Verification items for the finished model (mm, model axes). Face numbers are marked on the shaded views. Round coordinates to 2 decimals unless told otherwise and drop trailing zeros. Loops run counter-clockwise (first coordinate to the right, second up) from the corner with the lowest first, then second, coordinate; pieces in that order, holes last. Notation, with made-up numbers: (43, 70.5) - (48, 70.5) arc R27 ccw to (48, 92.5) - close; hole circle Ø9 at (-15.5, 72.5). An arc over 180 degrees is marked (long way). Use a Markdown table: item, result. Add a question column.
```python
from build123d import *

# Parameters (mm, degrees)
ESQUISSE1_W        = 39
ESQUISSE1_H        = 27
ESQUISSE1_W_2      = 33
ESQUISSE1_H_2      = 21
BOSS_EXTRU_1_DEPTH = 1.2
ESQUISSE2_W        = 39
ESQUISSE2_H        = 27
ESQUISSE2_W_2      = 36
ESQUISSE2_H_2      = 24
BOSS_EXTRU_3_DEPTH = 3.2
ESQUISSE3_W        = 39
ESQUISSE3_H        = 27
BOSS_EXTRU_4_DEPTH = 1.2
ESQUISSE5_R        = 6
BOSS_EXTRU_6_DEPTH = 20
ESQUISSE6_R        = 7.123023745
BOSS_EXTRU_7_DEPTH = 1.5
CONG_1_R           = 1.2


with BuildPart() as part:
    # Esquisse1 → Boss.-Extru.1 (new body)
    with BuildSketch(Plane(origin=(0, 0, 0), x_dir=(1, 0, 0), z_dir=(0, 1, 0))):
        with Locations((16.5, 10.5)):
            Rectangle(ESQUISSE1_W, ESQUISSE1_H)
        with Locations((16.5, 10.5)):
            Rectangle(ESQUISSE1_W_2, ESQUISSE1_H_2, mode=Mode.SUBTRACT)
    extrude(amount=BOSS_EXTRU_1_DEPTH)

    # Esquisse2 → Boss.-Extru.3 (add)
    with BuildSketch(Plane(origin=(0, 0, 0), x_dir=(-1, 0, 0), z_dir=(0, -1, 0))):
        with Locations((-16.5, 10.5)):
            Rectangle(ESQUISSE2_W, ESQUISSE2_H)
        with Locations((-16.5, 10.5)):
            Rectangle(ESQUISSE2_W_2, ESQUISSE2_H_2, mode=Mode.SUBTRACT)
    extrude(amount=BOSS_EXTRU_3_DEPTH)

    # Esquisse3 → Boss.-Extru.4 (add)
    with BuildSketch(Plane(origin=(0, -3.2, 0), x_dir=(-1, 0, 0), z_dir=(0, -1, 0))):
        with Locations((-16.5, 10.5)):
            Rectangle(ESQUISSE3_W, ESQUISSE3_H)
    extrude(amount=BOSS_EXTRU_4_DEPTH)

    # Esquisse5 → Boss.-Extru.6 (add)
    with BuildSketch(Plane(origin=(0, -4.4, 0), x_dir=(-1, 0, 0), z_dir=(0, -1, 0))):
        with Locations(Location((-16.5, 10.5, 0), (0, 0, 90))):
            Circle(ESQUISSE5_R)
    extrude(amount=BOSS_EXTRU_6_DEPTH)

    # Esquisse6 → Boss.-Extru.7 (add)
    with BuildSketch(Plane.XZ.offset(4.4)):
        with Locations(Location((16.5, -10.5, 0), (0, 0, 270))):
            Circle(ESQUISSE6_R)
    extrude(amount=BOSS_EXTRU_7_DEPTH)

    # Congé1
    # the kernel refuses this fillet: 1.2 mm, written as the material it takes off along each edge
    with BuildSketch(Plane(origin=(16.5, -5.9, -10.5), x_dir=(0, 0, -1), z_dir=(-1, 0, 0))) as cong_1_piece_1:
        with BuildLine():
            CenterArc((5.923023745, -1.197528562), CONG_1_R, 0, 86.32212933)
            Line((6, 0), (6.001539525, 0.023950571))
            ThreePointArc((6.001539525, 0.023950571), (6.561511873, 0.024), (7.123023745, 0.024))
            Line((7.123023745, 0.024), (7.147023745, 0))
            Line((7.147023745, 0), (7.147023745, -1.197528562))
            Line((7.147023745, -1.197528562), (7.123023745, -1.197528562))
        make_face()
    revolve(axis=Axis((16.5, -5.9, -10.5), (0, -1, 0)), mode=Mode.SUBTRACT)

    # Esquisse7 → Révolution2 (revolve)
    with BuildSketch(Plane.XZ.offset(24.4)):
        with BuildLine():
            Line((3.633416396, -7.841279791), (29.203795551, -12.548265009))
            ThreePointArc((29.203795551, -12.548265009), (14.065113365, -22.979961978), (3.633416396, -7.841279791))
        make_face()
    revolve(axis=Axis((3.633416396, -24.4, -7.841279791), (0.9834761213686738, 0, -0.181037892988263)))


solid = part.part
```
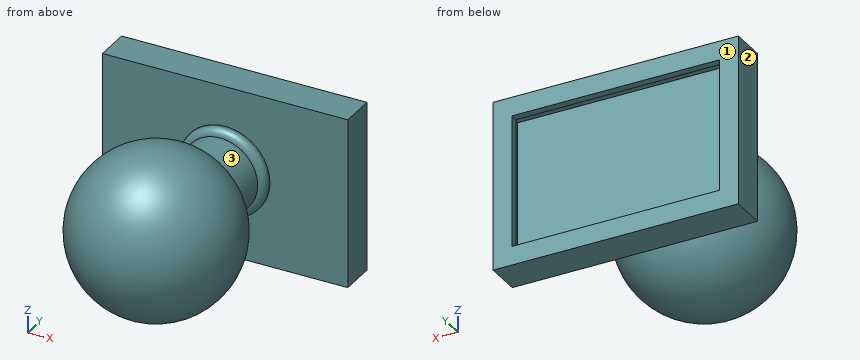
Q1. Go/stop test with flat-tipped pins: pin 1 Ø12 at (x, z) = (3, -2) entering from -Y; pin 2 Ø4 at (x, z) = (28.5, -13.5) entering from +Y; pin 3 Ø3 at (y, z) = (-29, -19.5) entering from +X. Record where each tip stops, or that it passes through.
Q2. Thickness scan on line 1 along X through (y, z) = (-1, -5); line 2 along Y through (x, z) = (-0.5, 0.25); line 3 along Y through (x, z) = (5, -19). Record the ranges inside material, lowest first.
Q3. Section check C-C on z = -20.5. Record the cut outline in (x, y).
Q4. Section check B-B on x = 27. Record the cut outline in (y, z).
Q5. Section check A-A on y = -2. Record the cut outline in (x, z).
Q6. Release check for a two-part mould opening along Y. For the marked faces 1, 2 and 3 record: +Y half, -Y half, draft (parallel to the pull), parting line (faces both ways), or undercut.
Q7. Section check D-D on x = 16.5. Record the cut outline in (y, z).
Determined:
| question | item | result |
|---|---|---|
| 1 | pin 1 | stops at y = -33.03 |
| 1 | pin 2 | stops at y = -3.2 |
| 1 | pin 3 | stops at x = 25.91 |
| 2 | line 1 | x = -3 to -1.5, 34.5 to 36 |
| 2 | line 2 | y = -4.4 to -3.2, 0 to 1.2 |
| 2 | line 3 | y = -4.4 to -3.2 |
| 3 | outline | (-3, -4.4) - (36, -4.4) - (36, 1.2) - (33, 1.2) - (33, 0) - (34.5, 0) - (34.5, -3.2) - (-1.5, -3.2) - (-1.5, 0) - (0, 0) - (0, 1.2) - (-3, 1.2) - close; circle Ø15.85 at (16.42, -24.4) |
| 4 | outline | circle Ø15.1 at (-24.4, -10.19); (-4.4, -24) - (1.2, -24) - (1.2, -21) - (0, -21) - (0, -22.5) - (-3.2, -22.5) - (-3.2, 1.5) - (0, 1.5) - (0, 0) - (1.2, 0) - (1.2, 3) - (-4.4, 3) - close |
| 5 | outline | (-3, -24) - (36, -24) - (36, 3) - (-3, 3) - close; hole (-1.5, -22.5) - (34.5, -22.5) - (34.5, 1.5) - (-1.5, 1.5) - close |
| 6 | face 1 | +Y half |
| 6 | face 2 | draft |
| 6 | face 3 | undercut |
| 7 | outline | (-13.03, -16.5) - (-5.9, -16.5) arc R1.2 ccw to (-4.7, -17.62) - (-4.4, -17.62) - (-4.4, -24) - (1.2, -24) - (1.2, -21) - (0, -21) - (0, -22.5) - (-3.2, -22.5) - (-3.2, 1.5) - (0, 1.5) - (0, 0) - (1.2, 0) - (1.2, 3) - (-4.4, 3) - (-4.4, -3.38) - (-4.7, -3.38) arc R1.2 ccw to (-5.9, -4.5) - (-12.71, -4.5) arc R13 ccw (long way) to start |
